```python
from build123d import *

# Parameters (mm, degrees)
F0_R      = 53
F1_DEPTH  = 26.5
F2_R      = 53
F2_R_2    = 48.75
F3_DEPTH  = 3.5
F4_R      = 2.75
F5_DEPTH  = 17
F6_DEPTH  = 4.5
F8_DEPTH  = 14
F9_R      = 3.25
F10_DEPTH = 12.5
F11_DEPTH = 10
F12_DEPTH = 22
F13_DEPTH = 5.5
F14_R     = 1.5
F15_DEPTH = 25
F16_R     = 1.5
F17_DEPTH = 25
F19_DEPTH = 2
F14_W     = 2
F14_H     = 5
F20_DEPTH = 2
F16_W     = 1
F16_H     = 5
F21_DEPTH = 2


with BuildPart() as f1:
    # F0 (on Top) → F1 (new body)
    with BuildSketch(Plane.XY):
        Circle(F0_R)
    extrude(amount=F1_DEPTH)

    # F2 (on face) → F3 (cut)
    with BuildSketch(Plane(origin=(0, 0, 0), x_dir=(1, 0, 0), z_dir=(0, 0, -1))):
        Circle(F2_R)
        Circle(F2_R_2, mode=Mode.SUBTRACT)
        with BuildLine():
            ThreePointArc((0, 6), (-4.2426406871, -4.2426406871), (6, 0))
            ThreePointArc((6, 0), (5.6381557247, 2.05212086), (4.5962666587, 3.8567256581))
            Line((4.5962666587, 3.8567256581), (0, 0))
            Line((0, 0), (0, 6))
        make_face()
        with BuildLine():
            Line((0, 0), (4.5962666587, 3.8567256581))
            ThreePointArc((4.5962666587, 3.8567256581), (2.5357095704, 5.4378467222), (0, 6))
            Line((0, 6), (0, 0))
        make_face()
    extrude(amount=-F3_DEPTH, mode=Mode.SUBTRACT)

    # F4 (on face) → F5 (cut)
    with BuildSketch(Plane(origin=(0, 0, 3.5), x_dir=(1, 0, 0), z_dir=(0, 0, -1))):
        Circle(F4_R)
    extrude(amount=-F5_DEPTH, mode=Mode.SUBTRACT)

    # F2 (on face) → F6 (cut)
    with BuildSketch(Plane(origin=(0, 0, 0), x_dir=(1, 0, 0), z_dir=(0, 0, -1))):
        with BuildLine():
            ThreePointArc((-40.25, 5.06e-08), (-35.0000000253, -5.25), (-29.75, 0))
            ThreePointArc((-29.75, 0), (-34.9999999747, 5.25), (-40.25, 5.06e-08))
        make_face()
        with BuildLine():
            ThreePointArc((40.25, 0), (35, -5.25), (29.75, 0))
            ThreePointArc((29.75, 0), (0, -29.75), (-29.75, 0))
            ThreePointArc((-29.75, 0), (-35.0000000253, -5.25), (-40.25, 5.06e-08))
            ThreePointArc((-40.25, 5.06e-08), (-2.53e-08, -40.25), (40.25, 0))
        make_face()
        with BuildLine():
            ThreePointArc((40.25, 0), (35, 5.25), (29.75, 0))
            ThreePointArc((29.75, 0), (35, -5.25), (40.25, 0))
        make_face()
    extrude(amount=-F6_DEPTH, mode=Mode.SUBTRACT)

    # F7 (on face) → F8 (cut)
    with BuildSketch(Plane.XY.offset(26.5)):
        with BuildLine():
            ThreePointArc((-9.5237930297, 1.6275609299), (-36.5712199238, -16.1753957641), (-4.7982329954, -9.9315291509))
            ThreePointArc((-4.7982329954, -9.9315291509), (-4.8174339562, -9.1357508964), (-4.8749921506, -8.3418247275))
            ThreePointArc((-4.8749921506, -8.3418247275), (-5.3803326375, -5.587516237), (-6.3441545093, -2.9583278322))
            ThreePointArc((-6.3441545093, -2.9583278322), (-7.7386969196, -0.529987713), (-9.5237930297, 1.6275609299))
        make_face()
    extrude(amount=-F8_DEPTH, mode=Mode.SUBTRACT)

    # F9 (on face) → F10 (cut)
    with BuildSketch(Plane.XY.offset(12.5)):
        with Locations((-21.2982329954, -9.9315291509)):
            Circle(F9_R)
    extrude(amount=-F10_DEPTH, mode=Mode.SUBTRACT)

    # F2 (on face) → F11 (cut)
    with BuildSketch(Plane(origin=(0, 0, 0), x_dir=(1, 0, 0), z_dir=(0, 0, -1))):
        with BuildLine():
            ThreePointArc((4.4625266318, 22.0827765885), (3.7995194773, 26.099690874), (1.8808305715, 29.6904862938))
            ThreePointArc((1.8808305715, 29.6904862938), (-10.1750992639, 27.9558554684), (-20.525476523, 21.5352574516))
            ThreePointArc((-20.525476523, 21.5352574516), (-7.763648091, 9.5857761597), (4.4625266318, 22.0827765885))
        make_face()
        with BuildLine():
            ThreePointArc((-20.525476523, 21.5352574516), (-10.1750992639, 27.9558554684), (1.8808305715, 29.6904862938))
            ThreePointArc((1.8808305715, 29.6904862938), (-12.3127251597, 33.8289343483), (-20.525476523, 21.5352574516))
        make_face()
        with BuildLine():
            ThreePointArc((13.2163960917, 26.6531306669), (5.8599977512, 18.0754756382), (8.4264888743, 7.0706637066))
            ThreePointArc((8.4264888743, 7.0706637066), (18.8184464785, 2.632197813), (28.5432128195, 8.3873417686))
            ThreePointArc((28.5432128195, 8.3873417686), (22.7898221828, 19.1229313882), (13.2163960917, 26.6531306669))
        make_face()
        with BuildLine():
            ThreePointArc((30.5020444133, 15.1055088276), (24.9457248488, 25.499512003), (13.2163960917, 26.6531306669))
            ThreePointArc((13.2163960917, 26.6531306669), (22.7898221828, 19.1229313882), (28.5432128195, 8.3873417686))
            ThreePointArc((28.5432128195, 8.3873417686), (30.0023486819, 11.6065522029), (30.5020444133, 15.1055088276))
        make_face()
    extrude(amount=-F11_DEPTH, mode=Mode.SUBTRACT)

    # F7 (on face) → F12 (join)
    with BuildSketch(Plane.XY.offset(26.5)):
        with BuildLine():
            Line((-48.4259152046, -28.0982647079), (-45.7069918435, -26.8304099227))
            ThreePointArc((-45.7069918435, -26.8304099227), (-48.0343127129, -22.3987678723), (-49.9331744609, -17.7673320523))
            Line((-49.9331744609, -17.7673320523), (-52.652097822, -19.0351868375))
            Line((-52.652097822, -19.0351868375), (-48.4259152046, -28.0982647079))
        make_face()
        with BuildLine():
            ThreePointArc((-13.3477590818, -51.2916886785), (-15.7549896718, -50.604152996), (-18.1270675963, -49.8037089017))
            ThreePointArc((-18.1270675963, -49.8037089017), (-20.458700255, -48.8921423531), (-22.7446852897, -47.8714872453))
            Line((-22.7446852897, -47.8714872453), (-23.7707457197, -50.6905651076))
            Line((-23.7707457197, -50.6905651076), (-14.3738195118, -54.1107665409))
            Line((-14.3738195118, -54.1107665409), (-13.3477590818, -51.2916886785))
        make_face()
        with BuildLine():
            ThreePointArc((43.6332188846, -30.0855814265), (42.1638253258, -32.1124871957), (40.6003554853, -34.0677433134))
            ThreePointArc((40.6003554853, -34.0677433134), (38.9462977901, -35.9469871956), (37.2053427877, -37.7460258577))
            Line((37.2053427877, -37.7460258577), (39.5034761171, -39.6743886867))
            Line((39.5034761171, -39.6743886867), (45.9313522139, -32.0139442555))
            Line((45.9313522139, -32.0139442555), (43.6332188846, -30.0855814265))
        make_face()
    extrude(amount=-F12_DEPTH)

    # F7 (on face) → F13 (cut)
    with BuildSketch(Plane.XY.offset(26.5)):
        with BuildLine():
            Line((-6.3517157751, 3.106724846), (-9.5237930297, 1.6275609299))
            ThreePointArc((-9.5237930297, 1.6275609299), (-7.7386969196, -0.529987713), (-6.3441545093, -2.9583278322))
            Line((-6.3441545093, -2.9583278322), (-4.0273153355, -1.8779679828))
            Line((-4.0273153355, -1.8779679828), (-6.3517157751, 3.106724846))
        make_face()
        with BuildLine():
            ThreePointArc((-6.3441545093, -2.9583278322), (-5.3803326375, -5.587516237), (-4.8749921506, -8.3418247275))
            Line((-4.8749921506, -8.3418247275), (-2.6602923891, -7.3090932683))
            Line((-2.6602923891, -7.3090932683), (-2.1493473528, -5.9052833183))
            Line((-2.1493473528, -5.9052833183), (-4.0273153355, -1.8779679828))
            Line((-4.0273153355, -1.8779679828), (-6.3441545093, -2.9583278322))
        make_face()
        Polygon((-2.1493473528, -5.9052833183), (-2.6602923891, -7.3090932683), (-1.7029148959, -6.8626608115), align=None)
    extrude(amount=-F13_DEPTH, mode=Mode.SUBTRACT)

    # F14 (on face) → F15 (cut)
    with BuildSketch(Plane(origin=(-19.0722826158, -52.4006658242, 0), x_dir=(0.9396926208, -0.3420201433, 0), z_dir=(-0.3420201433, -0.9396926208, 0))):
        with Locations((0, 7.5)):
            Circle(F14_R)
    extrude(amount=-F15_DEPTH, mode=Mode.SUBTRACT)

    # F16 (on face) → F17 (cut)
    with BuildSketch(Plane(origin=(42.7174141655, -35.8441664711, 0), x_dir=(0.6427876097, 0.7660444431, 0), z_dir=(0.7660444431, -0.6427876097, 0))):
        with Locations((0, 7.5)):
            Circle(F16_R)
    extrude(amount=-F17_DEPTH, mode=Mode.SUBTRACT)

    # F18 (on face) → F19 (join)
    with BuildSketch(Plane(origin=(-50.5390065133, -23.5667257727, 0), x_dir=(0.4226182617, -0.906307787, 0), z_dir=(-0.906307787, -0.4226182617, 0))):
        Polygon((2, 19.5), (-2, 19.5), (-2, 18.5), (-0.5, 18.5), (-0.5, 14.5), (-2, 14.5), (-2, 13.5), (2, 13.5), (2, 14.5), (0.5, 14.5), (0.5, 18.5), (2, 18.5), align=None)
    extrude(amount=F19_DEPTH)

    # F14 (on face) → F20 (join)
    with BuildSketch(Plane(origin=(-19.0722826158, -52.4006658242, 0), x_dir=(0.9396926208, -0.3420201433, 0), z_dir=(-0.3420201433, -0.9396926208, 0))):
        Polygon((3, 20), (-3, 20), (-3, 19), (-2, 19), (-2, 14), (-3, 14), (-3, 13), (3, 13), (3, 14), (2, 14), (2, 19), (3, 19), align=None)
        with Locations((0, 16.5)):
            Rectangle(F14_W, F14_H, mode=Mode.SUBTRACT)
    extrude(amount=F20_DEPTH)

    # F16 (on face) → F21 (join)
    with BuildSketch(Plane(origin=(42.7174141655, -35.8441664711, 0), x_dir=(0.6427876097, 0.7660444431, 0), z_dir=(0.7660444431, -0.6427876097, 0))):
        Polygon((3.25, 20), (-3.25, 20), (-3.25, 19), (-2.5, 19), (-2.5, 14), (-3.25, 14), (-3.25, 13), (3.25, 13), (3.25, 14), (2.5, 14), (2.5, 19), (3.25, 19), align=None)
        with Locations((-1, 16.5)):
            Rectangle(F16_W, F16_H, mode=Mode.SUBTRACT)
        with Locations((1, 16.5)):
            Rectangle(F16_W, F16_H, mode=Mode.SUBTRACT)
    extrude(amount=F21_DEPTH)


solid = f1.part
```
Input: part model. Units: mm. Frame: model coordinates. A direction names the side the tool comes from. Round coordinates to 2 decimals unless told otherwise and drop trailing zeros. Order: outer loops, then holes, each group sorted by start corner. A loop starts at its lowest first (then second) coordinate and runs counter-clockwise, first axis right, second up. Notation, with made-up numbers: (2, -18) - (8, -18) arc R30 cw to (8, 17) - close; hole circle Ø5 at (85.5, 34.5). An arc over 180 degrees is marked (long way). One line per question, with ' | ' between items. Start each with the question number.
1) Cut plane D-D, the plane x = -35. Return the cut outline in (y, z).
2) Cut plane B-B, the plane y = 38.5. Return the cut outline in (x, z), then the cut area to 3 significant figures.
3) Contact query for flat-ended pins moving along their axis: P1, Ø2, axis at x = 45.5, y = -34.5, coming from the +Z side; P2, Ø1.9, axis at x = -21, y = -50.5, coming from the -Z side; P3, Ø12.5, axis at x = -12.5, y = -19, coming from the -Z side. Output: stop coordinate, or through.
4) Ray query, probe 1 along X at (y, z) = (-16, 9.5); probe 2 along X at (y, z) = (0, 16.5); probe 3 along Y at (x, z) = (0, 12.75). Return the intervals inside material, ascending.
5) Pull-direction query (X, two-part tool) for faces 6 (the flat face through (-52.36, -24.39, 16.54)), 7 (the cylindrical face through (35.12, -5.25, 2.22)), 8 (the flat face through (-19, -53, 13)); classes: +X half, -X half, draft (parallel to the pull), parting line (faces both ways), or undercut.
6) Cut plane C-C, the plane x = 17. Return the cut outline in (y, z), then the cut area to 3 significant figures.
7) Set-up query: faces 1 (the flat face through (-19, -53, 19)), 2 (the flat face through (-7.916, 2.377, 23.788)), 3 (the cylindrical face through (-34.88, -5.25, 2.22)), 4 (the flat face through (-51, -24, 19.5)), 5 (the flat face through (-51.27, -18.39, 15.65)). Return all of +Z, -Z, +X, -X, +Y, -Y with unobstructed straight access to the full face (end or side cutting, diameter ignored); none if empty.
8) Cut plane A-A, the plane z = 24. Return the cut outline in (x, y) (3 decimals), then the cut area to 3 significant figures.
Worked out:
1) outline: (-39.8, 3.5) - (-33.93, 3.5) - (-33.93, 0) - (-5.25, 0) - (-5.25, 4.5) - (19.88, 4.5) - (19.88, 0) - (33.93, 0) - (33.93, 3.5) - (39.8, 3.5) - (39.8, 26.5) - (-0.74, 26.5) - (-0.74, 12.5) - (-19.12, 12.5) - (-19.12, 26.5) - (-39.8, 26.5) - close
2) outline: (-36.42, 3.5) - (-29.91, 3.5) - (-29.91, 0) - (-11.74, 0) - (-11.74, 4.5) - (11.74, 4.5) - (11.74, 0) - (29.91, 0) - (29.91, 3.5) - (36.42, 3.5) - (36.42, 26.5) - (-36.42, 26.5) - close | area: 1,780 mm^2
3) P1: stops at z = 20 | P2: stops at z = 4.5 | P3: stops at z = 10
4) probe 1: x = -50.53 to -18.96, 2.88 to 5.53, 30.47 to 50.53 | probe 2: x = -53 to -34.47, -8.12 to -2.75, 2.75 to 53 | probe 3: y = -53 to -2.75, 2.75 to 53
5) face 6: -X half | face 7: undercut | face 8: draft
6) outline: (-50.2, 3.5) - (-45.69, 3.5) - (-45.69, 0) - (-27.57, 0) - (-27.57, 10) - (-2.65, 10) - (-2.65, 0) - (24.41, 0) - (24.41, 4.5) - (36.48, 4.5) - (36.48, 0) - (45.69, 0) - (45.69, 3.5) - (50.2, 3.5) - (50.2, 26.5) - (-50.2, 26.5) - close | area: 2,330 mm^2
7) face 1: none | face 2: +Z | face 3: -Z | face 4: +Z, -X, -Y | face 5: +Z, -Z, -X
8) outline: (-52.652, -19.035) - (-48.426, -28.098) - (-45.707, -26.83) arc R53 ccw to (-22.745, -47.871) - (-23.771, -50.691) - (-14.374, -54.111) - (-13.348, -51.292) arc R53 ccw to (37.205, -37.746) - (39.503, -39.674) - (45.931, -32.014) - (43.633, -30.086) arc R53 ccw (long way) to (-49.933, -17.767) - close; hole (-9.524, 1.628) arc R16.5 ccw (long way) to (-4.875, -8.342) - (-1.703, -6.863) - (-6.352, 3.107) - close | area: 8,020 mm^2
